Job drawing, mm, ordinate dimensions from the low corner. One solid piece. A direction names the side the tool comes from. Round coordinates to 2 decimals unless told otherwise and drop trailing zeros. Loops run counter-clockwise (first coordinate to the right, second up) from the corner with the lowest first, then second, coordinate; pieces in that order, holes last.
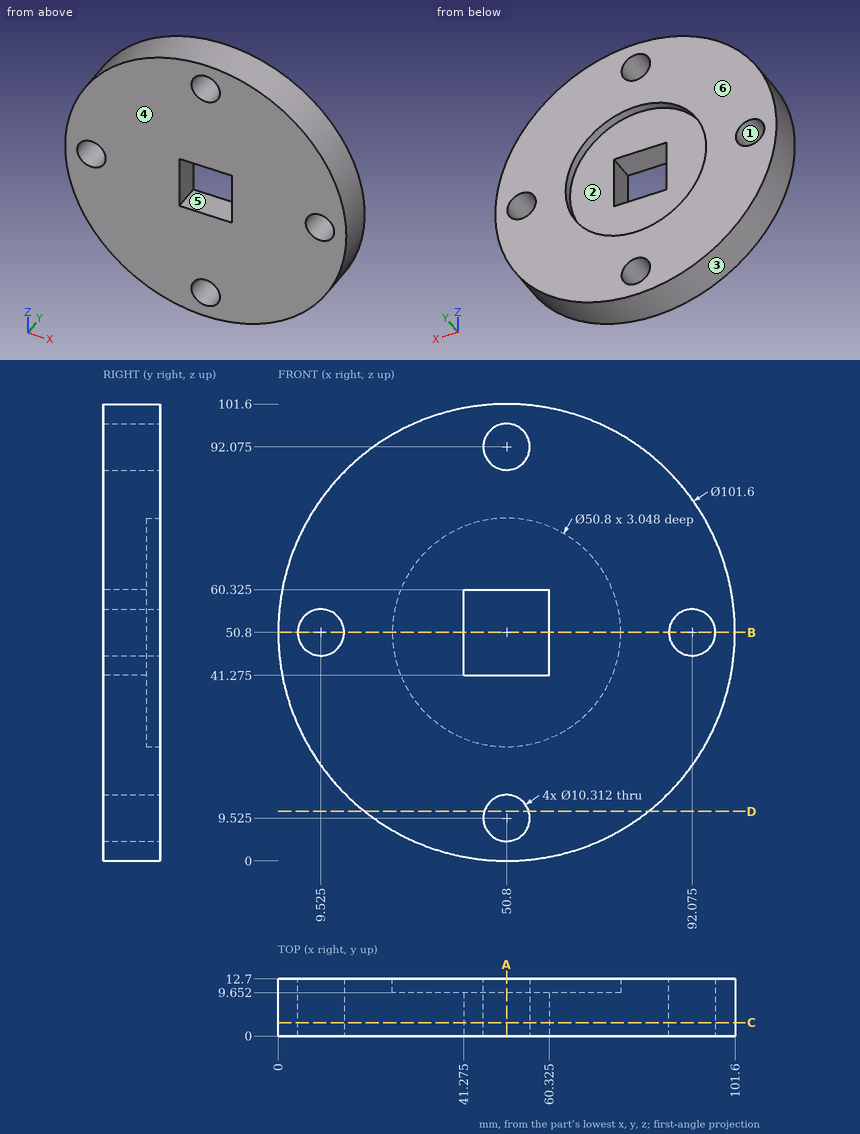
Item 1: Cut at B-B, the plane z = 50.8. Give the cut face in (x, y) (1 decimal).
Answers follow:
outline: (0, 0) - (4.4, 0) - (4.4, 12.7) - (0, 12.7) - close; (14.7, 0) - (41.3, 0) - (41.3, 9.7) - (25.4, 9.7) - (25.4, 12.7) - (14.7, 12.7) - close; (60.3, 0) - (86.9, 0) - (86.9, 12.7) - (76.2, 12.7) - (76.2, 9.7) - (60.3, 9.7) - close; (97.2, 0) - (101.6, 0) - (101.6, 12.7) - (97.2, 12.7) - close
Item 2: Flat gauge pins, fed straight in: P1, Ø2, axis at y = 5.5, z = 10.5, coming from the +X side; P2, Ø6, axis at y = 6.5, z = 74.5, coming from the -X side. Where does each tip first touch, or does it go through?
Answers follow:
P1: stops at x = 82.99
P2: stops at x = 4.41
Item 3: Cut at A-A, the plane x = 50.8. Give the cut face in (y, z) (1 decimal).
Answers follow:
outline: (0, 0) - (12.7, 0) - (12.7, 4.4) - (0, 4.4) - close; (0, 14.7) - (12.7, 14.7) - (12.7, 25.4) - (9.7, 25.4) - (9.7, 41.3) - (0, 41.3) - close; (0, 60.3) - (9.7, 60.3) - (9.7, 76.2) - (12.7, 76.2) - (12.7, 86.9) - (0, 86.9) - close; (0, 97.2) - (12.7, 97.2) - (12.7, 101.6) - (0, 101.6) - close
Item 4: Two-plate mould, pull along Z, no slides. Class the marked faces 1, 2, 3 and 4: released by +Z, released by -Z, zero draft, split by the parting line, or undercut.
Answers follow:
face 1: undercut
face 2: undercut
face 3: split by the parting line
face 4: zero draft
Item 5: Cut at C-C, the plane y = 3. Give the cut face in (x, z) (1 decimal), plus the area to 3 significant figures.
Answers follow:
outline: circle Ø101.6 at (50.8, 50.8); hole circle Ø10.3 at (9.5, 50.8); hole (41.3, 41.3) - (60.3, 41.3) - (60.3, 60.3) - (41.3, 60.3) - close; hole circle Ø10.3 at (50.8, 9.5); hole circle Ø10.3 at (50.8, 92.1); hole circle Ø10.3 at (92.1, 50.8)
area: 7,410 mm2
Item 6: Probe line 1 (Z direction, x = 50.8, y = 5.25) (1 decimal); line 2 (Z direction, x = 50.8, y = 11.15); line 3 (Y direction, x = 37.5, z = 69.5). List the from-to ranges inside material, lowest first.
Answers follow:
line 1: z = 0 to 4.4, 14.7 to 41.3, 60.3 to 86.9, 97.2 to 101.6
line 2: z = 0 to 4.37, 14.68 to 25.4, 76.2 to 86.92, 97.23 to 101.6
line 3: y = 0 to 9.65
Item 7: 3-axis set-ups, long thin cutter, end or side, ignore diameter. For the marked faces 5 and 6: which of +Z, -Z, +X, -X, +Y, -Y reach the whole face in a straight line?
Answers follow:
face 5: +Y, -Y
face 6: +Z, -Z, +X, -X, +Y
Item 8: Cut at D-D, the plane z = 11. Give the cut face in (x, y), plus the area to 3 significant figures.
Answers follow:
outline: (19.23, 0) - (45.86, 0) - (45.86, 12.7) - (19.23, 12.7) - close; (55.74, 0) - (82.37, 0) - (82.37, 12.7) - (55.74, 12.7) - close
area: 676 mm2
